from build123d import *

# Parameters (mm, degrees)
SKETCH_W        = 32
SKETCH_H        = 30
PAD_DEPTH       = 8.75
SKETCH001_W     = 28
SKETCH001_H     = 26
POCKET_DEPTH    = 6.75
SKETCH002_R     = 1
SKETCH002_R_2   = 0.5
PAD001_DEPTH    = 2.75
SKETCH003_W     = 26
SKETCH003_H     = 6.75
POCKET001_DEPTH = 2
SKETCH004_W     = 8
SKETCH004_H     = 6.75
PAD002_DEPTH    = 6
SKETCH005_R     = 3.375
SKETCH005_R_2   = 1.5
PAD003_DEPTH    = 8
SKETCH006_R     = 1.5
POCKET002_DEPTH = 8


with BuildPart() as part:
    # Sketch → Pad (new body)
    with BuildSketch(Plane.XY):
        with Locations((16, 15)):
            Rectangle(SKETCH_W, SKETCH_H)
    extrude(amount=PAD_DEPTH)

    # Sketch001 (on Face6 of Pad) → Pocket (cut)
    with BuildSketch(Plane.XY.offset(8.75)):
        with Locations((16, 15)):
            Rectangle(SKETCH001_W, SKETCH001_H)
    extrude(amount=-POCKET_DEPTH, mode=Mode.SUBTRACT)

    # Sketch002 (on Face11 of Pocket) → Pad001 (join)
    with BuildSketch(Plane.XY.offset(2)):
        with Locations((5.6, 26)):
            Circle(SKETCH002_R)
        with Locations((5.6, 26)):
            Circle(SKETCH002_R_2, mode=Mode.SUBTRACT)
        with Locations((26.4, 26)):
            Circle(SKETCH002_R)
        with Locations((26.4, 26)):
            Circle(SKETCH002_R_2, mode=Mode.SUBTRACT)
        with Locations((26.05, 13.715)):
            Circle(SKETCH002_R)
        with Locations((26.05, 13.715)):
            Circle(SKETCH002_R_2, mode=Mode.SUBTRACT)
        with Locations((5.6, 13.645)):
            Circle(SKETCH002_R)
        with Locations((5.6, 13.645)):
            Circle(SKETCH002_R_2, mode=Mode.SUBTRACT)
    extrude(amount=PAD001_DEPTH)

    # Sketch003 (on Face1 of Pad001) → Pocket001 (cut)
    with BuildSketch(Plane.XZ):
        with Locations((16, 5.375)):
            Rectangle(SKETCH003_W, SKETCH003_H)
    extrude(amount=-POCKET001_DEPTH, mode=Mode.SUBTRACT)

    # Sketch004 (on Face9 of Pocket001) → Pad002 (join)
    with BuildSketch(Plane(origin=(0, 30, 0), x_dir=(-1, 0, 0), z_dir=(0, 1, 0))):
        with Locations((-20, 3.375)):
            Rectangle(SKETCH004_W, SKETCH004_H)
    extrude(amount=PAD002_DEPTH)

    # Sketch005 (on Face19 of Pad002) → Pad003 (join)
    with BuildSketch(Plane(origin=(16, 0, 0), x_dir=(0, -1, 0), z_dir=(-1, 0, 0))):
        with Locations((-36, 3.375)):
            Circle(SKETCH005_R)
        with Locations((-36, 3.375)):
            Circle(SKETCH005_R_2, mode=Mode.SUBTRACT)
    extrude(amount=-PAD003_DEPTH)

    # Sketch006 (on Face34 of Pad003) → Pocket002 (cut)
    with BuildSketch(Plane(origin=(16, 0, 0), x_dir=(0, -1, 0), z_dir=(-1, 0, 0))):
        with Locations((-35.974457, 3.342444)):
            Circle(SKETCH006_R)
    extrude(amount=-POCKET002_DEPTH, mode=Mode.SUBTRACT)


solid = part.part
Here's how the part is built. I have some questions about the finished solid (model axes, mm). A direction names the side the tool comes from. Coordinates: 2 decimals unless noted, no trailing zeros. Loops run counter-clockwise (first coordinate to the right, second up) from the corner with the lowest first, then second, coordinate; pieces in that order, holes last.
1. I need wall thicknesses on L1, parallel to Y at x = 5.6, z = 3 (3 decimals); L2, parallel to X at y = 15.5, z = 4.5; L3, parallel to Y at x = 26.05, z = 3.95 (3 decimals). Which ranges of each line are inside material? Lowest first, please.
2. Imagine slicing it at B-B, the plane y = 4.5. Please give me the cut outline in (x, z), and give its area (3 significant figures).
3. Imagine slicing it at D-D, the plane x = 9. Please give me the cut outline in (y, z), and give its area (3 significant figures).
4. If we mould it in two halves opening along Z, with no side actions, what happens to faces 5 (the flat face through (5.6, 26, 2)), 6 (the flat face through (0, 15, 4)), 7 (the cylindrical face through (19.944, 34.644, 2.65)), 8 (the flat face through (16, 14, 0))? For each: pulls with the +Z half, pulls with the -Z half, needs draft (parallel to the pull), parting line crosses it, or undercut.
5. For faces 1 (the flat face through (16, 34, 3)), 2 (the cylindrical face through (19.944, 37.343, 4.043)), 3 (the flat face through (30, 15, 5)), 4 (the flat face through (5, 14, 4.75)), which set-ups out of +Z, -Z, +X, -X, +Y, -Y let a thin tool reach every point of the face, with its end or its side?
6. For P1, Ø5, axis at y = 35.97, z = 3.34, coming from the -X side; P2, Ø14, axis at x = 18, y = 9, coming from the +Z side; P3, Ø1.1, axis at x = 29.5, z = 6, coming from the +Y side, each with a flat end and sliding along its axis, tell me the tip position at first contact or that it passes through.
7. Imagine slicing it at C-C, the plane x = 18. Please give me the cut outline in (y, z) (3 decimals).
8. Imagine slicing it at A-A, the plane z = 3.5. Count the separate pieces of the cut face and the enclosed holes in it, and give its area (3 significant figures).
Taken from the geometry:
1. L1: y = 12.645 to 13.145, 14.145 to 14.645, 25 to 25.5, 26.5 to 27, 28 to 30
1. L2: x = 0 to 2, 30 to 32
1. L3: y = 12.715 to 13.215, 14.215 to 14.715, 25.063 to 25.643, 26.357 to 26.937, 28 to 30
2. outline: (0, 0) - (32, 0) - (32, 8.75) - (30, 8.75) - (30, 2) - (2, 2) - (2, 8.75) - (0, 8.75) - close
2. area: 91.0 mm2
3. outline: (0, 0) - (30, 0) - (30, 8.75) - (28, 8.75) - (28, 2) - (0, 2) - close
3. area: 73.5 mm2
4. face 5: pulls with the +Z half
4. face 6: needs draft
4. face 7: undercut
4. face 8: pulls with the -Z half
5. face 1: +Z, -Z, -X, +Y
5. face 2: +X, -X
5. face 3: +Z
5. face 4: +Z, -Y
6. P1: stops at x = 16
6. P2: stops at z = 2
6. P3: stops at y = 30
7. outline: (0, 0) - (36, 0) arc R3.375 ccw to (36, 6.75) - (30, 6.75) - (30, 8.75) - (28, 8.75) - (28, 2) - (0, 2) - close; hole (36, 4.842) arc R1.5 ccw (long way) to (37.167, 2.433) arc R1.5 ccw to (36, 4.875) - close
8. separate pieces: 6
8. enclosed holes: 4
8. area: 240 mm2
